```python
from build123d import *

# Parameters (mm, degrees)
F2_R      = 8.4836
F3_DEPTH  = 32.893
F2_R_2    = 6.096
F4_DEPTH  = 15.621
F5_DEPTH  = 25.4
F6_R      = 6.096
F7_DEPTH  = 5.588
F9_DEPTH  = 25.4
F10_DEPTH = 4.064


with BuildPart() as f1:
    # F0 (on Front) → F1 (revolve)
    with BuildSketch(Plane.XZ):
        with BuildLine():
            Line((-32.766, 0), (0, 0))
            Line((0, 0), (0, 9.525))
            Line((0, 9.525), (-32.766, 9.525))
            Line((-32.766, 9.525), (-32.766, 7.1613881737))
            Line((-32.766, 7.1613881737), (-18.1468881737, 7.1613881737))
            ThreePointArc((-18.1468881737, 7.1613881737), (-15.748, 4.7625), (-18.1468881737, 2.3636118263))
            Line((-18.1468881737, 2.3636118263), (-32.766, 2.3636118263))
            Line((-32.766, 2.3636118263), (-32.766, 0))
        make_face()
    revolve(axis=Axis((0, 0, 13.9041366056), (0, 0, 1)))

    # F2 (on Top) → F3 (join)
    with BuildSketch(Plane.XY):
        with BuildLine():
            Line((-11.6078, -1.8505721543), (-14.6153072736, -1.8505721543))
            ThreePointArc((-14.6153072736, -1.8505721543), (-14.2560030009, -3.7145931726), (-13.659986963, -5.5169357592))
            Line((-13.659986963, -5.5169357592), (-4.8393499563, -10.6095329094))
            Line((-4.8393499563, -10.6095329094), (-6.3803690894, -13.2786563433))
            ThreePointArc((-6.3803690894, -13.2786563433), (-4.2668294637, -14.1005670215), (-2.052186963, -14.5883636049))
            Line((-2.052186963, -14.5883636049), (6.7684500437, -9.4957664547))
            Line((6.7684500437, -9.4957664547), (8.3094691767, -12.1648898886))
            ThreePointArc((8.3094691767, -12.1648898886), (10.0780345166, -10.7454662199), (11.6078, -9.0714278457))
            Line((11.6078, -9.0714278457), (11.6078, 1.1137664547))
            Line((11.6078, 1.1137664547), (14.6898382661, 1.1137664547))
            ThreePointArc((14.6898382661, 1.1137664547), (14.3448639802, 3.3551008016), (13.659986963, 5.5169357592))
            Line((13.659986963, 5.5169357592), (4.8393499563, 10.6095329094))
            Line((4.8393499563, 10.6095329094), (6.3803690894, 13.2786563433))
            ThreePointArc((6.3803690894, 13.2786563433), (4.2668294637, 14.1005670215), (2.052186963, 14.5883636049))
            Line((2.052186963, 14.5883636049), (-5.8039, 10.052649682))
            Line((-5.8039, 10.052649682), (-6.7684500437, 9.4957664547))
            Line((-6.7684500437, 9.4957664547), (-8.3094691767, 12.1648898886))
            ThreePointArc((-8.3094691767, 12.1648898886), (-10.0780345166, 10.7454662199), (-11.6078, 9.0714278457))
            Line((-11.6078, 9.0714278457), (-11.6078, 0))
            Line((-11.6078, 0), (-11.6078, -1.8505721543))
        make_face()
        Circle(F2_R, mode=Mode.SUBTRACT)
    extrude(amount=F3_DEPTH)

    # F2 (on Top) → F4 (join)
    with BuildSketch(Plane.XY):
        Circle(F2_R)
        Circle(F2_R_2, mode=Mode.SUBTRACT)
    extrude(amount=F4_DEPTH)

    # F2 (on Top) → F5 (cut)
    with BuildSketch(Plane.XY):
        Circle(F2_R_2)
    extrude(amount=F5_DEPTH, mode=Mode.SUBTRACT)

    # F6 (on face) → F7 (join)
    with BuildSketch(Plane(origin=(0, 0, 0), x_dir=(1, 0, 0), z_dir=(0, 0, -1))):
        with BuildLine():
            Line((-8.0137, 1.9177), (-8.0137, -8.3625714986))
            ThreePointArc((-8.0137, -8.3625714986), (-5.1960588966, -10.3514714752), (-1.9177, -11.4225398432))
            Line((-1.9177, -11.4225398432), (-1.9177, -8.0137))
            Line((-1.9177, -8.0137), (8.3625714986, -8.0137))
            ThreePointArc((8.3625714986, -8.0137), (10.3514714752, -5.1960588966), (11.4225398432, -1.9177))
            Line((11.4225398432, -1.9177), (8.0137, -1.9177))
            Line((8.0137, -1.9177), (8.0137, 8.3625714986))
            ThreePointArc((8.0137, 8.3625714986), (5.1960588966, 10.3514714752), (1.9177, 11.4225398432))
            Line((1.9177, 11.4225398432), (1.9177, 8.0137))
            Line((1.9177, 8.0137), (-8.3625714986, 8.0137))
            ThreePointArc((-8.3625714986, 8.0137), (-10.3514714752, 5.1960588966), (-11.4225398432, 1.9177))
            Line((-11.4225398432, 1.9177), (-8.0137, 1.9177))
        make_face()
        Circle(F6_R, mode=Mode.SUBTRACT)
    extrude(amount=F7_DEPTH)

    # F8 (on face) → F9 (cut)
    with BuildSketch(Plane.XY.offset(9.525)):
        with BuildLine():
            ThreePointArc((-8.1849360794, 20.1539266654), (-6.9739301336, 12.0260401102), (-0.0684106271, 16.4805743843))
            ThreePointArc((-0.0684106271, 16.4805743843), (-1.2729957626, 19.6943902925), (-4.293224081, 21.3246844208))
            ThreePointArc((-4.293224081, 21.3246844208), (-6.3664785516, 21.1627903823), (-8.1849360794, 20.1539266654))
        make_face()
    extrude(amount=-F9_DEPTH, mode=Mode.SUBTRACT)

    # F8 (on face) → F10 (cut)
    with BuildSketch(Plane.XY.offset(9.525)):
        with BuildLine():
            ThreePointArc((-8.1849360794, 20.1539266654), (-6.3664785516, 21.1627903823), (-4.293224081, 21.3246844208))
            Line((-4.293224081, 21.3246844208), (-7.4752096352, 31.90191212))
            ThreePointArc((-7.4752096352, 31.90191212), (-9.4392344031, 31.3769279867), (-11.3669216335, 30.7311543645))
            Line((-11.3669216335, 30.7311543645), (-8.1849360794, 20.1539266654))
        make_face()
    extrude(amount=-F10_DEPTH, mode=Mode.SUBTRACT)


solid = f1.part
```
Verification items for the finished model (mm, model axes). A direction names the side the tool comes from. Coordinates: 2 decimals unless noted, no trailing zeros. Loops run counter-clockwise (first coordinate to the right, second up) from the corner with the lowest first, then second, coordinate; pieces in that order, holes last. Notation, with made-up numbers: (16, 72) - (32, 72) arc R27 ccw to (32, 96) - close; hole circle Ø4 at (-20, -2.75). An arc over 180 degrees is marked (long way). Put each result on its own line as item: value.
Item 1: Scan lines: line 1 along Z through (x, y) = (-15, -23.5) (3 decimals); line 2 along X through (y, z) = (10.5, 21); line 3 along X through (y, z) = (0, 5). Record each from-to range of solid material in increasing order.
Conclusion:
line 1: z = 0 to 2.364, 7.161 to 9.525
line 2: x = -10.33 to -7.35, -5.03 to 5.03
line 3: x = -15.76 to -6.1, 6.1 to 15.76
Item 2: Gauge pin test, flat ends, axial feed: pin 1 Ø12 at (x, z) = (11, 16.5) entering from +Y; pin 2 Ø4.5 at (x, z) = (-2, -3) entering from -Y; pin 3 Ø3.5 at (y, z) = (1.5, 19) entering from -X; pin 4 Ø6 at (x, y) = (-4.96, 16.48) entering from -Z. Record the tip position at first contact, or that the pin passes through.
Conclusion:
pin 1: stops at y = 13.86
pin 2: stops at y = -8.01
pin 3: stops at x = -11.61
pin 4: passes through
Item 3: Section check D-D (y = 23.5). Enter the section's corners in (x, z) (3 decimals).
Conclusion:
outline: (-22.833, 0) - (22.833, 0) - (22.833, 2.364) - (-22.833, 2.364) - close; (-22.833, 7.161) - (-9.192, 7.161) - (-9.192, 9.525) - (-22.833, 9.525) - close; (-4.948, 7.161) - (22.833, 7.161) - (22.833, 9.525) - (-4.948, 9.525) - close
Item 4: Section check A-A (z = -2). Enter the section's corners in (x, y), then the cut area to 3 significant figures.
Conclusion:
outline: (-11.42, -1.92) arc R11.58 ccw to (-8.36, -8.01) - (1.92, -8.01) - (1.92, -11.42) arc R11.58 ccw to (8.01, -8.36) - (8.01, 1.92) - (11.42, 1.92) arc R11.58 ccw to (8.36, 8.01) - (-1.92, 8.01) - (-1.92, 11.42) arc R11.58 ccw to (-8.01, 8.36) - (-8.01, -1.92) - close; hole circle Ø12.19 at (0, 0)
area: 195 mm2
Item 5: Draft check along X on faces 1 (the face through (-0.794, -6.044, 5.165)), 2 (the face through (-5.24, 10.33, -2.75)), 3 (the face through (3, 8.014, -3)). Enter one of: pulls with the +X half, pulls with the -X half, needs draft (parallel to the pull), parting line crosses it, or undercut.
Conclusion:
face 1: undercut
face 2: pulls with the -X half
face 3: needs draft
Item 6: Section check B-B (y = 0). Enter the section's corners in (x, z) (1 decimal).
Conclusion:
outline: (-32.8, 0) - (-8, 0) - (-8, -5.6) - (-6.1, -5.6) - (-6.1, 15.6) - (-8.5, 15.6) - (-8.5, 32.9) - (-11.6, 32.9) - (-11.6, 9.5) - (-32.8, 9.5) - (-32.8, 7.2) - (-18.1, 7.2) arc R2.4 cw to (-18.1, 2.4) - (-32.8, 2.4) - close; (6.1, -5.6) - (8, -5.6) - (8, 0) - (32.8, 0) - (32.8, 2.4) - (18.1, 2.4) arc R2.4 cw to (18.1, 7.2) - (32.8, 7.2) - (32.8, 9.5) - (11.6, 9.5) - (11.6, 32.9) - (8.5, 32.9) - (8.5, 15.6) - (6.1, 15.6) - close
Item 7: Section check C-C (x = -19.5). Enter the section's corners in (y, z) (3 decimals), then the cut area to 3 significant figures.
Conclusion:
outline: (-26.332, 0) - (26.332, 0) - (26.332, 2.364) - (-26.332, 2.364) - close; (-26.332, 7.161) - (26.332, 7.161) - (26.332, 9.525) - (-26.332, 9.525) - close
area: 249 mm2
Item 8: Set-up check for faces 4 (the face through (8.014, -3, -3)), 5 (the face through (-11.608, 4, 21)), 6 (the face through (1.918, -10, -3)): record each of +Z, -Z, +X, -X, +Y, -Y from which the full face is reachable in a straight line by a thin tool's end or side.
Conclusion:
face 4: -Z, +X, -Y
face 5: +Z, -X, +Y
face 6: -Z, -X, -Y
